Here's how the part is built. I have some questions about the finished solid (model axes, mm). A direction names the side the tool comes from. Round coordinates to 2 decimals unless told otherwise and drop trailing zeros. Write each loop counter-clockwise with the first axis right and the second up, starting at its lowest first coordinate (ties: lowest second). Pieces come first, ordered by that corner, then holes. Notation, with made-up numbers: (-8, 81.25) -> (8, 81.25) arc R21 cw to (8, 115.25) -> close; hole circle Ø6 at (63.25, -24.75). An arc over 180 degrees is marked (long way). Answer as CSV lines item,"result".
from build123d import *

# Parameters (mm, degrees)
F0_W     = 43.4
F0_H     = 43.4
F0_R     = 3
F0_R_2   = 16
F1_DEPTH = 17.5
F3_R     = 16
F3_R_2   = 14
F4_DEPTH = 2
F5_R     = 3


with BuildPart() as f1:
    # F0 (on Front) → F1 (new body, symmetric)
    with BuildSketch(Plane.XZ):
        Rectangle(F0_W, F0_H)
        with Locations((-16.5, -16.5)):
            Circle(F0_R, mode=Mode.SUBTRACT)
        with Locations((16.5, -16.5)):
            Circle(F0_R, mode=Mode.SUBTRACT)
        with Locations((-16.5, 16.5)):
            Circle(F0_R, mode=Mode.SUBTRACT)
        Circle(F0_R_2, mode=Mode.SUBTRACT)
        with Locations((16.5, 16.5)):
            Circle(F0_R, mode=Mode.SUBTRACT)
    extrude(amount=F1_DEPTH, both=True)

    # F3 (on offset) → F4 (join)
    with BuildSketch(Plane(origin=(0, 14.75, 0), x_dir=(-1, 0, 0), z_dir=(0, 1, 0))):
        Circle(F3_R)
        Circle(F3_R_2, mode=Mode.SUBTRACT)
    extrude(amount=-F4_DEPTH)

    # F5
    f5_edges = [f1.edges().sort_by_distance(p)[0] for p in [
        (-21.7, 0, 21.7),
        (21.7, 0, 21.7),
        (21.7, 0, -21.7),
        (-21.7, 0, -21.7),
    ]]
    fillet(f5_edges, radius=F5_R)


solid = f1.part
Item 1: Will this pin go through, and if not, where does the flat tip stop? pin 1 (16 mm diameter, centred on x = -1, z = 0, fed in from -Y).
Results found:
pin 1,"passes through"
Item 2: Suppose I cut it at B-B, the plane z = 5. List the corners of the cut face in (x, y) for me, then the cut area to 3 significant figures.
Results found:
outline,"(-21.7, -17.5) -> (-15.2, -17.5) -> (-15.2, 12.75) -> (-13.08, 12.75) -> (-13.08, 14.75) -> (-15.2, 14.75) -> (-15.2, 17.5) -> (-21.7, 17.5) -> close; (13.08, 12.75) -> (15.2, 12.75) -> (15.2, -17.5) -> (21.7, -17.5) -> (21.7, 17.5) -> (15.2, 17.5) -> (15.2, 14.75) -> (13.08, 14.75) -> close"
area,"464 mm²"
Item 3: If we mould it in two halves opening along X, with no side actions, what happens to faces 4 (the cylindrical face through (-20.8, 0.25, 20.84)), 5 (the cylindrical face through (15.85, 0.25, -19.43)), 6 (the cylindrical face through (-3.47, 16.14, -15.62)), 7 (the flat face through (9, 17.5, -14))? For each: pulls with the +X half, pulls with the -X half, needs draft (parallel to the pull), parting line crosses it, or undercut.
Results found:
face 4,"pulls with the -X half"
face 5,"undercut"
face 6,"undercut"
face 7,"needs draft"
Item 4: Suppose I cut it at D-D, the plane x = -17. List the corners of the cut face in (y, z) for me.
Results found:
outline,"(-17.5, -21.7) -> (17.5, -21.7) -> (17.5, -19.46) -> (-17.5, -19.46) -> close; (-17.5, -13.54) -> (17.5, -13.54) -> (17.5, 13.54) -> (-17.5, 13.54) -> close; (-17.5, 19.46) -> (17.5, 19.46) -> (17.5, 21.7) -> (-17.5, 21.7) -> close"
Item 5: I need wall thicknesses on L1, parallel to Z at x = -16.5, y = -14; L2, parallel to Z at x = 0, y = 14.25; L3, parallel to X at y = 16.1, z = 0. Which ranges of each line are inside material? Lowest first, please.
Results found:
L1,"z = -21.7 to -19.5, -13.5 to 13.5, 19.5 to 21.7"
L2,"z = -21.7 to -14, 14 to 21.7"
L3,"x = -21.7 to -16, 16 to 21.7"
Item 6: For faces 1 (the flat face through (0.07, 14.75, -14.15)), 2 (the cylindrical face through (-18.9, 0.2, 14.7)), 3 (the flat face through (0.07, 12.75, -14.15)), which set-ups out of +Z, -Z, +X, -X, +Y, -Y let a thin tool reach every point of the face, with its end or its side?
Results found:
face 1,"+Y"
face 2,"+Y, -Y"
face 3,"-Y"
Item 7: Suppose I cut it at A-A, the plane x = 0. List the corners of the cut face in (y, z) for me.
Results found:
outline,"(-17.5, -21.7) -> (17.5, -21.7) -> (17.5, -16) -> (14.75, -16) -> (14.75, -14) -> (12.75, -14) -> (12.75, -16) -> (-17.5, -16) -> close; (-17.5, 16) -> (12.75, 16) -> (12.75, 14) -> (14.75, 14) -> (14.75, 16) -> (17.5, 16) -> (17.5, 21.7) -> (-17.5, 21.7) -> close"
Item 8: Suppose I cut it at C-C, the plane y = -3.5. List the corners of the cut face in (x, z) for me.
Results found:
outline,"(-21.7, -18.7) arc R3 ccw to (-18.7, -21.7) -> (18.7, -21.7) arc R3 ccw to (21.7, -18.7) -> (21.7, 18.7) arc R3 ccw to (18.7, 21.7) -> (-18.7, 21.7) arc R3 ccw to (-21.7, 18.7) -> close; hole circle Ø6 at (-16.5, -16.5); hole circle Ø6 at (-16.5, 16.5); hole circle Ø32 at (0, 0); hole circle Ø6 at (16.5, -16.5); hole circle Ø6 at (16.5, 16.5)"
